Model file for the job. Use its own axes, mm. A direction names the side the tool comes from. Give positions to 0.01 mm unless a question says otherwise; leave off trailing zeros. Loops run counter-clockwise (first coordinate to the right, second up) from the corner with the lowest first, then second, coordinate; pieces in that order, holes last. Notation, with made-up numbers: M 79.5,58 L 131.5,58 A22 ccw 131.5,71 Z; hole C 38.25,1.5 d4. An arc over 180 degrees is marked long. Use CSV: the item, a comma, the result in double quotes. Start each with the question number.
(1) Two-plate mould, pull along X, no slides. Class faces 4 (the face through (95, -2, -118.808)), 5 (the face through (33.538, -1.565, -60.4)): pulls with the +X half, pulls with the -X half, needs draft (parallel to the pull), parting line crosses it, or undercut.
(2) Wall check: line 1 along Z through (x, y) = (92, -1.8); line 2 along X through (y, z) = (-2.45, 8); line 3 along X through (y, z) = (-0.15, -93). Give the ranges that are in metal, low to high. Write a range as from..to.
(3) Slice it at C-C on z = -5.5. List the corners of the cut face in (x, y) (3 decimals).
(4) Tool access for faces 1 (the face through (19, -2, 0)), 2 (the face through (42, 0, -66)), 3 (the face through (2, -2, 0)): list every direction of +Z, -Z, +X, -X, +Y, -Y with a clear straight run to the whole face (end or side of a thin tool).
(5) Flat gauge pins, fed straight in: P1, Ø8, axis at x = 38.5, z = -99, coming from the +Y side; P2, Ø1.5, axis at y = -1.5, z = -117, coming from the +X side (3 decimals); P3, Ø1, axis at y = -2, z = 9.5, coming from the +X side. Where does each tip first touch, or does it go through?
(6) Slice it at A-A on x = 87. List the corners of the cut face in (y, z) (3 decimals), and give its area (3 significant figures).
(7) Slice it at B-B on y = -1.45. State how many separate pieces and enclosed holes the cut face has, and give its area (3 significant figures).
```python
from build123d import *

# Parameters (mm, degrees)
BOSS_EXTRUDE1_DEPTH = 3.175


with BuildPart() as part:
    # Sketch1 → Boss-Extrude1 (new body)
    with BuildSketch(Plane(origin=(0, 0, 0), x_dir=(1, 0, 0), z_dir=(0, 1, 0))):
        Polygon((98.425, 127), (98.425, 118.8085), (92.075, 118.8085), (92.075, 115.8875), (98.425, 115.8875), (98.425, 107.95), (63.697477915, 107.95), (20.517477915, 0), (16.610957915, 0), (16.610957915, -15.875), (3.90652, -15.875), (3.90652, 0), (0, 0), (50.8, 127), align=None)
        Polygon((74.356304753, 123.754225326), (72.787834938, 119.633813496), (68.38440659, 119.415387337), (71.818467282, 116.65040662), (70.665468711, 112.395), (74.356304753, 114.806559768), (78.047140796, 112.395), (76.894142225, 116.65040662), (80.328202917, 119.415387337), (75.924774569, 119.633813496), align=None, mode=Mode.SUBTRACT)
        Polygon((47.649827384, 99.756946391), (46.081357569, 95.636534562), (41.67792922, 95.418108402), (45.111989912, 92.653127685), (43.958991341, 88.397721065), (47.649827384, 90.809280833), (51.340663426, 88.397721065), (50.187664855, 92.653127685), (53.621725547, 95.418108402), (49.218297199, 95.636534562), align=None, mode=Mode.SUBTRACT)
        Polygon((32.742653477, 62.489011624), (31.174183662, 58.368599795), (26.770755314, 58.150173636), (30.204816006, 55.385192919), (29.051817435, 51.129786299), (32.742653477, 53.541346066), (36.433489519, 51.129786299), (35.280490948, 55.385192919), (38.71455164, 58.150173636), (34.311123292, 58.368599795), align=None, mode=Mode.SUBTRACT)
        Polygon((17.261423317, 23.785936225), (15.692953502, 19.665524395), (11.289525154, 19.447098236), (14.723585846, 16.682117519), (13.570587275, 12.426710899), (17.261423317, 14.838270667), (20.952259359, 12.426710899), (19.799260788, 16.682117519), (23.23332148, 19.447098236), (18.829893132, 19.665524395), align=None, mode=Mode.SUBTRACT)
    extrude(amount=-BOSS_EXTRUDE1_DEPTH)


solid = part.part
```
Reply:
1,face 4,"needs draft"
1,face 5,"undercut"
2,line 1,"z = -127..-107.95"
2,line 2,"x = 3.91..16.61"
2,line 3,"x = 37.2..44.68, 50.62..57.72"
3,outline,"M 2.2,-3.175 L 22.717,-3.175 L 22.717,0 L 2.2,0 Z"
4,face 1,"+Z, +X, +Y, -Y"
4,face 2,"+Z, -Z, +X, -X, +Y"
4,face 3,"+Z, -X, +Y, -Y"
5,P1,"stops at y = 0"
5,P2,"stops at x = 92.075"
5,P3,"stops at x = 16.61"
6,outline,"M -3.175,-127 L 0,-127 L 0,-107.95 L -3.175,-107.95 Z"
6,area,"60.5 mm^2"
7,separate pieces,"1"
7,enclosed holes,"4"
7,area,"3,180 mm^2"
